Model file for the job. Use its own axes, mm. Face numbers are marked on the shaded views. A direction names the side the tool comes from. Coordinates: 2 decimals unless noted, no trailing zeros. Order: outer loops, then holes, each group sorted by start corner. A loop starts at its lowest first (then second) coordinate and runs counter-clockwise, first axis right, second up. Notation, with made-up numbers: (-36, 63) -> (7, 63) arc R27 cw to (7, 97) -> close; hole circle Ø4 at (-7.5, -5.75). An arc over 180 degrees is marked (long way). Use CSV: the item, a comma, the result in double quotes. Start each with the question number.
(1) Pin check, flat tips, straight feed: pin 1 Ø1 at (x, y) = (72, -6.5) entering from +Z; pin 2 Ø11 at (x, z) = (265, -18.5) entering from -Y; pin 3 Ø6.5 at (x, z) = (288.5, -19.5) entering from -Y; pin 4 Ø22 at (x, y) = (31.5, -25) entering from -Z. Stop position of each tip, or through.
(2) Tool access for the marked faces 1, 2 and 3: list every direction of +Z, -Z, +X, -X, +Y, -Y with a clear straight run to the whole face (end or side of a thin tool).
(3) Cut at D-D on x = 11.5. Write the cut outline in (y, z).
(4) Pull direction X, two halves, no side cores. Call the marked faces 4, 5, 6 and 7: pulls with the +X half, pulls with the -X half, needs draft (parallel to the pull), parting line crosses it, or undercut.
(5) Cut at A-A on z = -181.5. Write the cut outline in (x, y), plus the area to 3 significant figures.
(6) Cut at B-B on x = 74. Write the cut outline in (y, z).
(7) Cut at C-C on z = -133.5. Write the cut outline in (x, y), plus the area to 3 significant figures.
(8) Probe L1, parallel to Y at x = 257, z = -277; L2, parallel to Z at x = 270, y = -29; L3, parallel to X at y = -12, z = -207. List the from-to ranges inside material, lowest first.
```python
from build123d import *

# Parameters (mm, degrees)
F1_DEPTH  = 50
F3_DEPTH  = 333
F4_T      = -4
F5_R      = 6
F6_DEPTH  = 302.7
F7_R      = 20
F9_START  = 20
F8_R      = 15
F8_R_2    = 11.2
F9_DEPTH  = 25
F10_START = 27
F8_R_3    = 8
F10_DEPTH = 11
F11_DEPTH = 117.9
F12_DEPTH = 24
F14_START = 20
F13_R     = 6.5
F13_R_2   = 4
F14_DEPTH = 15


with BuildPart() as f1:
    # F0 (on Front) → F1 (new body)
    with BuildSketch(Plane.XZ):
        Polygon((300, 0), (0, 0), (0, -177), (40, -177), (40, -300), (260, -300), (260, -177), (300, -177), align=None)
    extrude(amount=F1_DEPTH)

    # F2 (on Right) → F3 (cut)
    with BuildSketch(Plane.YZ):
        Polygon((0, 0), (-20, 0), (-20, -60), (0, -100), align=None)
    extrude(amount=F3_DEPTH, mode=Mode.SUBTRACT)

    # F4
    f4_openings = [f1.faces().sort_by_distance(p)[0] for p in [
        (150, -50, -139.136228),
    ]]
    offset(amount=F4_T, openings=f4_openings, kind=Kind.INTERSECTION)

    # F5 (on Right) → F6 (cut)
    with BuildSketch(Plane.YZ):
        with BuildLine():
            ThreePointArc((-7.8504098361, -275.2528829848), (-7.7751231532, -276.125), (-7.75, -277))
            ThreePointArc((-7.75, -277), (-7.7751231532, -277.875), (-7.8504098361, -278.7471170152))
            ThreePointArc((-7.8504098361, -278.7471170152), (-6.5485877504, -278.2724419855), (-6, -277))
            ThreePointArc((-6, -277), (-6.5485877504, -275.7275580145), (-7.8504098361, -275.2528829848))
        make_face()
        with BuildLine():
            ThreePointArc((-16.9382526366, -263.0065115535), (-15.375, -263.7931125923), (-13.9121571995, -264.7536285687))
            ThreePointArc((-13.9121571995, -264.7536285687), (-13.6983254787, -264.2943735518), (-13.625, -263.7931125923))
            ThreePointArc((-13.625, -263.7931125923), (-14.9707674642, -262.0904393832), (-16.9382526366, -263.0065115535))
        make_face()
        with BuildLine():
            ThreePointArc((-7.8504098361, -278.7471170152), (-7.7751231532, -277.875), (-7.75, -277))
            ThreePointArc((-7.75, -277), (-7.7751231532, -276.125), (-7.8504098361, -275.2528829848))
            ThreePointArc((-7.8504098361, -275.2528829848), (-9.5, -277), (-7.8504098361, -278.7471170152))
        make_face()
        with BuildLine():
            ThreePointArc((-16.9382526366, -263.0065115535), (-16.25, -265.3086570489), (-13.9121571995, -264.7536285687))
            ThreePointArc((-13.9121571995, -264.7536285687), (-15.375, -263.7931125923), (-16.9382526366, -263.0065115535))
        make_face()
        with BuildLine():
            ThreePointArc((-32.0878428005, -264.7536285687), (-30.625, -263.7931125923), (-29.0617473634, -263.0065115535))
            ThreePointArc((-29.0617473634, -263.0065115535), (-31.5, -262.2775681357), (-32.0878428005, -264.7536285687))
        make_face()
        with BuildLine():
            ThreePointArc((-28.875, -263.7931125923), (-28.9223267909, -263.3888800565), (-29.0617473634, -263.0065115535))
            ThreePointArc((-29.0617473634, -263.0065115535), (-30.625, -263.7931125923), (-32.0878428005, -264.7536285687))
            ThreePointArc((-32.0878428005, -264.7536285687), (-30.1237390405, -265.4697871136), (-28.875, -263.7931125923))
        make_face()
        with BuildLine():
            ThreePointArc((-38.1495901639, -278.7471170152), (-38.25, -277), (-38.1495901639, -275.2528829848))
            ThreePointArc((-38.1495901639, -275.2528829848), (-40, -277), (-38.1495901639, -278.7471170152))
        make_face()
        with BuildLine():
            ThreePointArc((-36.5, -277), (-36.9775580145, -275.7985877504), (-38.1495901639, -275.2528829848))
            ThreePointArc((-38.1495901639, -275.2528829848), (-38.25, -277), (-38.1495901639, -278.7471170152))
            ThreePointArc((-38.1495901639, -278.7471170152), (-36.9775580145, -278.2014122496), (-36.5, -277))
        make_face()
        with BuildLine():
            ThreePointArc((-32.0878428005, -289.2463714313), (-31.5, -291.7224318643), (-29.0617473634, -290.9934884465))
            ThreePointArc((-29.0617473634, -290.9934884465), (-30.625, -290.2068874077), (-32.0878428005, -289.2463714313))
        make_face()
        with BuildLine():
            ThreePointArc((-32.0878428005, -289.2463714313), (-30.625, -290.2068874077), (-29.0617473634, -290.9934884465))
            ThreePointArc((-29.0617473634, -290.9934884465), (-28.9223267909, -290.6111199435), (-28.875, -290.2068874077))
            ThreePointArc((-28.875, -290.2068874077), (-30.1237390405, -288.5302128864), (-32.0878428005, -289.2463714313))
        make_face()
        with BuildLine():
            ThreePointArc((-13.625, -290.2068874077), (-13.6983254787, -289.7056264482), (-13.9121571995, -289.2463714313))
            ThreePointArc((-13.9121571995, -289.2463714313), (-15.375, -290.2068874077), (-16.9382526366, -290.9934884465))
            ThreePointArc((-16.9382526366, -290.9934884465), (-14.9707674642, -291.9095606168), (-13.625, -290.2068874077))
        make_face()
        with BuildLine():
            ThreePointArc((-16.9382526366, -290.9934884465), (-15.375, -290.2068874077), (-13.9121571995, -289.2463714313))
            ThreePointArc((-13.9121571995, -289.2463714313), (-16.25, -288.6913429511), (-16.9382526366, -290.9934884465))
        make_face()
        with Locations((-23, -277)):
            Circle(F5_R)
    extrude(amount=F6_DEPTH, mode=Mode.SUBTRACT)

    # F7
    f7_edges = [f1.edges().sort_by_distance(p)[0] for p in [
        (300, -25, -177),
        (296, -27, -173),
        (4, -27, -173),
        (0, -25, -177),
        (300, -35, 0),
        (296, -37, -4),
        (0, -35, 0),
        (4, -37, -4),
    ]]
    fillet(f7_edges, radius=F7_R)

    # F8 (on Front) → F9 (join)
    with BuildSketch(Plane.XZ.offset(F9_START)):
        with Locations((40, -20)):
            Circle(F8_R)
        with Locations((40, -20)):
            Circle(F8_R_2, mode=Mode.SUBTRACT)
        with Locations((260, -20)):
            Circle(F8_R)
        with Locations((260, -20)):
            Circle(F8_R_2, mode=Mode.SUBTRACT)
    extrude(amount=F9_DEPTH)

    # F8 (on Front) → F10 (join)
    with BuildSketch(Plane.XZ.offset(F10_START)):
        with Locations((40, -20)):
            Circle(F8_R_2)
        with Locations((40, -20)):
            Circle(F8_R_3, mode=Mode.SUBTRACT)
        with Locations((260, -20)):
            Circle(F8_R_2)
        with Locations((260, -20)):
            Circle(F8_R_3, mode=Mode.SUBTRACT)
    extrude(amount=F10_DEPTH)

    # F8 (on Front) → F11 (cut)
    with BuildSketch(Plane.XZ):
        with Locations((40, -20)):
            Circle(F8_R_3)
        with Locations((260, -20)):
            Circle(F8_R_3)
    extrude(amount=F11_DEPTH, mode=Mode.SUBTRACT)

    # F8 (on Front) → F12 (cut)
    with BuildSketch(Plane.XZ):
        with Locations((40, -20)):
            Circle(F8_R_2)
        with Locations((40, -20)):
            Circle(F8_R_3, mode=Mode.SUBTRACT)
        with Locations((260, -20)):
            Circle(F8_R_2)
        with Locations((260, -20)):
            Circle(F8_R_3, mode=Mode.SUBTRACT)
    extrude(amount=F12_DEPTH, mode=Mode.SUBTRACT)

    # F13 (on Front) → F14 (join)
    with BuildSketch(Plane.XZ.offset(F14_START)):
        with Locations((288.5, -19.5)):
            Circle(F13_R)
        with Locations((288.5, -19.5)):
            Circle(F13_R_2, mode=Mode.SUBTRACT)
        with Locations((11.5, -19.5)):
            Circle(F13_R)
        with Locations((11.5, -19.5)):
            Circle(F13_R_2, mode=Mode.SUBTRACT)
    extrude(amount=F14_DEPTH)


solid = f1.part
```
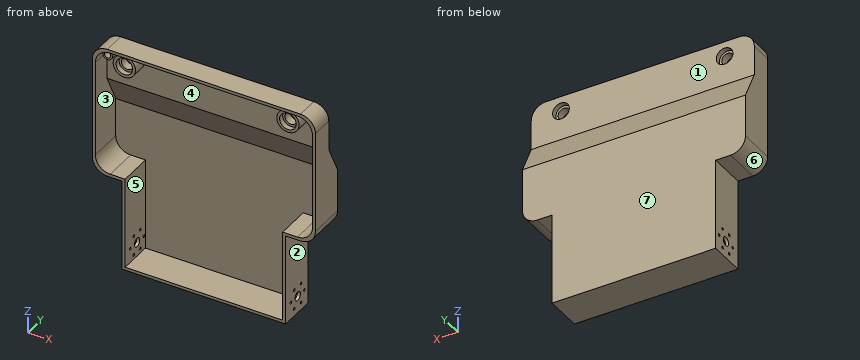
Outcome:
1,pin 1,"z = -86"
1,pin 2,"y = -38"
1,pin 3,"y = -24"
1,pin 4,"z = -300"
2,face 1,"+Z, +X, -X, +Y"
2,face 2,"-Z, +X, +Y, -Y"
2,face 3,"-Y"
3,outline,"(-50, -175.1) -> (0, -175.1) -> (0, -100) -> (-20, -60) -> (-20, -1.9) -> (-50, -1.9) -> (-50, -8.39) -> (-24, -8.39) -> (-24, -13) -> (-35, -13) -> (-35, -15.5) -> (-24, -15.5) -> (-24, -23.5) -> (-35, -23.5) -> (-35, -26) -> (-24, -26) -> (-24, -60.94) -> (-4, -100.94) -> (-4, -168.61) -> (-50, -168.61) -> close"
4,face 4,"undercut"
4,face 5,"undercut"
4,face 6,"pulls with the -X half"
4,face 7,"needs draft"
5,outline,"(40, -50) -> (44, -50) -> (44, -4) -> (256, -4) -> (256, -50) -> (260, -50) -> (260, 0) -> (40, 0) -> close"
5,area,"1,250 mm2"
6,outline,"(-50, -300) -> (0, -300) -> (0, -100) -> (-20, -60) -> (-20, 0) -> (-50, 0) -> (-50, -4) -> (-24, -4) -> (-24, -60.94) -> (-4, -100.94) -> (-4, -296) -> (-50, -296) -> close"
7,outline,"(0, -50) -> (4, -50) -> (4, -4) -> (296, -4) -> (296, -50) -> (300, -50) -> (300, 0) -> (0, 0) -> close"
7,area,"1,570 mm2"
8,L1,"-50 to -40, -36.5 to -29, -17 to -9.5, -6 to 0"
8,L2,"-177 to -173, -31.18 to -8.82, -4 to 0"
8,L3,"40 to 44, 256 to 260"
